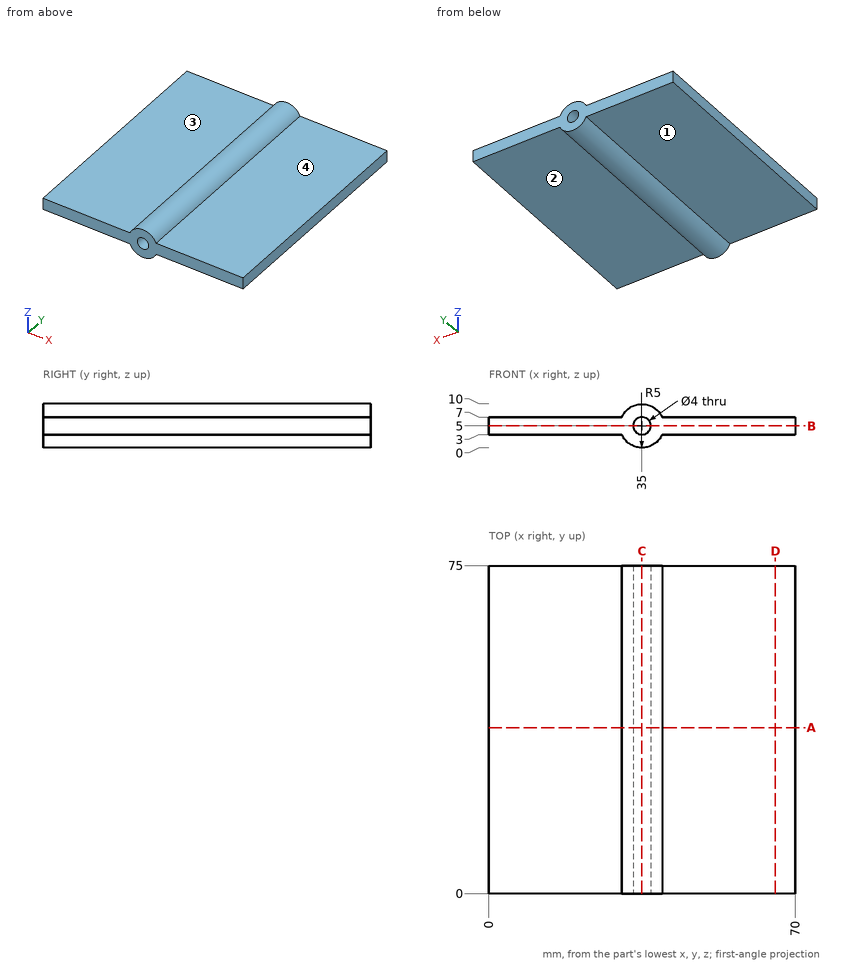
Geometry: see drawing. Coordinates: mm, zero at the bounding-box minimum. A direction names the side the tool comes from. Coordinates: 2 decimals unless noted, no trailing zeros. Loops run counter-clockwise (first coordinate to the right, second up) from the corner with the lowest first, then second, coordinate; pieces in that order, holes last. Notation, with made-up numbers: M -25,57.5 L 6,57.5 A31 cw 6,94.5 Z; hole C 44.5,34 d8. An arc over 180 degrees is marked long. Answer in a Markdown table with one row per item.
1. Material intervals for line 1 (X direction, y = 52.5, z = 5); line 2 (Z direction, x = 35, y = 57); line 3 (Z direction, x = 26, y = 35), sorted ascending.
Response:
| item | result |
|---|---|
| line 1 | x = 0 to 33, 37 to 70 |
| line 2 | z = 0 to 3, 7 to 10 |
| line 3 | z = 3 to 7 |
2. Reachability of the marked faces 1, 2, 3 and 4 from +Z, -Z, +X, -X, +Y, -Y: full face, straight path, thin tool, end or side. Return the list, or none.
Response:
| item | result |
|---|---|
| face 1 | -Z, -X, +Y, -Y |
| face 2 | -Z, +X, +Y, -Y |
| face 3 | +Z, -X, +Y, -Y |
| face 4 | +Z, +X, +Y, -Y |
3. Section B-B, the plane z = 5. Output: boundary loops of the cut face in (x, y).
Response:
| item | result |
|---|---|
| outline | M 0,0 L 33,0 L 33,75 L 0,75 Z; M 37,0 L 70,0 L 70,75 L 37,75 Z |
4. Section C-C, the plane x = 35. Output: boundary loops of the cut face in (y, z).
Response:
| item | result |
|---|---|
| outline | M 0,0 L 75,0 L 75,3 L 0,3 Z; M 0,7 L 75,7 L 75,10 L 0,10 Z |
5. First-contact query: pin 1 (10 mm diameter, centred on x = 41, y = 60.5, fed in from +Z); pin 2 (1 mm diameter, centred on x = 11.5, y = 56, fed in from +Z); pin 3 (15 mm diameter, centred on x = 11, y = 37.5, fed in from -Z). Flat tips, straight axial feed; report the tip coordinate or a pass-through.
Response:
| item | result |
|---|---|
| pin 1 | stops at z = 9.9 |
| pin 2 | stops at z = 7 |
| pin 3 | stops at z = 3 |
6. Section A-A, the plane y = 38. Output: boundary loops of the cut face in (x, z).
Response:
| item | result |
|---|---|
| outline | M 0,3 L 30.42,3 A5 ccw 39.58,3 L 70,3 L 70,7 L 39.58,7 A5 ccw 30.42,7 L 0,7 Z; hole C 35,5 d4 |
7. Section D-D, the plane x = 65.5. Output: boundary loops of the cut face in (y, z), then the cut area to 3 significant figures.
Response:
| item | result |
|---|---|
| outline | M 0,3 L 75,3 L 75,7 L 0,7 Z |
| area | 300 mm2 |
